from build123d import *

# Parameters (mm, degrees)
SKETCH_1_R               = 2.5
SKETCH_1_R_2             = 0.925
EXTRUDE_1_DEPTH          = 3
CUT_EXTRUDE_2_DEPTH      = 5.636809248
PATTERN_CIRCULAR_1_COUNT = 6
EXTRUDE_START            = 1
SKETCH_2_R               = 2.5
EXTRUDE_2_DEPTH          = 1
SKETCH_2_3_W             = 4
SKETCH_2_3_H             = 0.6
EXTRUDE_3_DEPTH          = 2
SKETCH_2_4_W             = 0.6
SKETCH_2_4_H             = 2.5
EXTRUDE_4_DEPTH          = 1


with BuildPart() as part:
    # 草图1 → 凸台-拉伸1 (new body)
    with BuildSketch(Plane.XY):
        Circle(SKETCH_1_R)
        Circle(SKETCH_1_R_2, mode=Mode.SUBTRACT)
    extrude(amount=EXTRUDE_1_DEPTH)

    # 草图1<3> → 切除-拉伸2 (cut, through all)
    with BuildSketch(Plane.XY):
        with BuildLine():
            Line((1.03720071, 0.442455292), (0.85081958, 0.362947713))
            ThreePointArc((0.85081958, 0.362947713), (0.906265169, 0.185225388), (0.925, 0))
            ThreePointArc((0.925, 0), (0.906265169, -0.185225388), (0.85081958, -0.362947713))
            Line((0.85081958, -0.362947713), (1.03720071, -0.442455292))
            add(Edge.make_bspline(
                [(1.03720071, -0.442455292), (1.04510701, -0.445828009), (1.067871965, -0.453596987), (1.113314547, -0.461522157), (1.188023144, -0.464138789), (1.284367459, -0.452433849), (1.404657298, -0.420054467), (1.538436606, -0.361310704), (1.660601931, -0.285147073), (1.748638649, -0.214154324), (1.79986288, -0.166729965), (1.818980117, -0.1481092)],
                knots=[0, 0, 0, 0, 0, 0.005604068, 0.015718248, 0.029959916, 0.048733667, 0.068727063, 0.096888892, 0.125050566, 0.14248965, 0.14248965, 0.14248965, 0.14248965, 0.14248965], degree=4))
            ThreePointArc((1.818980117, -0.1481092), (1.823494408, -0.074115744), (1.825, 0))
            ThreePointArc((1.825, 0), (1.823494408, 0.074115744), (1.818980117, 0.1481092))
            add(Edge.make_bspline(
                [(1.03720071, 0.442455292), (1.04510701, 0.445828009), (1.067871965, 0.453596987), (1.113314547, 0.461522157), (1.188023144, 0.464138789), (1.284367459, 0.452433849), (1.404657298, 0.420054467), (1.538436606, 0.361310704), (1.660601931, 0.285147073), (1.748638649, 0.214154324), (1.79986288, 0.166729965), (1.818980117, 0.1481092)],
                knots=[0, 0, 0, 0, 0, 0.005604068, 0.015718248, 0.029959916, 0.048733667, 0.068727063, 0.096888892, 0.125050566, 0.14248965, 0.14248965, 0.14248965, 0.14248965, 0.14248965], degree=4))
        make_face()
    cut_extrude_2 = extrude(amount=CUT_EXTRUDE_2_DEPTH, mode=Mode.SUBTRACT)

    # 阵列(圆周)1: 切除-拉伸2 ×6 about axis
    pattern_circular_1_axis = Axis((0, 0, 3), (0, 0, 1))
    for i in range(1, PATTERN_CIRCULAR_1_COUNT):
        add(cut_extrude_2.rotate(pattern_circular_1_axis, i * 360 / PATTERN_CIRCULAR_1_COUNT), mode=Mode.SUBTRACT)

    # 草图2 → 凸台-拉伸2 (add)
    with BuildSketch(Plane(origin=(0, 0, 0), x_dir=(-1, 0, 0), z_dir=(0, 0, -1)).offset(EXTRUDE_START)):
        Circle(SKETCH_2_R)
    extrude(amount=-EXTRUDE_2_DEPTH)

    # 草图2<3> → 凸台-拉伸3 (add)
    with BuildSketch(Plane(origin=(0, 0, 0), x_dir=(-1, 0, 0), z_dir=(0, 0, -1)).offset(EXTRUDE_START)):
        Rectangle(SKETCH_2_3_W, SKETCH_2_3_H)
    extrude(amount=EXTRUDE_3_DEPTH)

    # 草图2<4> → 凸台-拉伸4 (add)
    with BuildSketch(Plane(origin=(0, 0, 0), x_dir=(-1, 0, 0), z_dir=(0, 0, -1)).offset(EXTRUDE_START)):
        Rectangle(SKETCH_2_4_W, SKETCH_2_4_H)
    extrude(amount=EXTRUDE_4_DEPTH)


solid = part.part
Geometry: final body of the model. Coordinates: model frame, mm. A direction names the side the tool comes from. Round coordinates to 2 decimals unless told otherwise and drop trailing zeros. Loops run counter-clockwise (first coordinate to the right, second up) from the corner with the lowest first, then second, coordinate; pieces in that order, holes last. Notation, with made-up numbers: (73.25, 60.25) -> (91.25, 60.25) arc R22 cw to (91.25, 98.25) -> close; hole circle Ø8 at (3.25, 19.25). An arc over 180 degrees is marked (long way). One line per question, with ' | ' between items. Start each with the question number.
1. Mould query, pull axis X, two halves, no side actions, for faces 4 (the face through (0, -0.3, -2.2)), 5 (the face through (-0.3, 0.8, -1.5)), 6 (the face through (0, 0, 0)). Classes: pulls with the +X half, pulls with the -X half, needs draft (parallel to the pull), parting line crosses it, or undercut.
2. Contact query for flat-ended pins moving along their axis: pin 1 (0.8 mm diameter, centred on y = -1, z = -1.5, fed in from +X); pin 2 (1.6 mm diameter, centred on x = -1, z = -1.5, fed in from +Y); pin 3 (0.5 mm diameter, centred on y = 0, z = -1.5, fed in from +X). Output: stop coordinate, or through.
3. Set-up query: faces 1 (the face through (0.3, -0.8, -1.5)), 2 (the face through (-0.3, -0.8, -1.5)), 3 (the face through (0.3, 0.8, -1.5)). Return all of +Z, -Z, +X, -X, +Y, -Y with unobstructed straight access to the full face (end or side cutting, diameter ignored); none if empty.
4. Section A-A on x = 0. Output: boundary loops of the cut face in (y, z) (3 decimals).
5. Line query: line 1 along X through (y, z) = (1.25, 2); line 2 along Z through (x, y) = (-0.6, -1); line 3 along Z through (x, y) = (-1.4, -1.05). Output: solid intervals per line, ascending. Write a range as [from, to].
Returned:
1) face 4: needs draft | face 5: pulls with the -X half | face 6: undercut
2) pin 1: stops at x = 0.3 | pin 2: stops at y = 2.47 | pin 3: stops at x = 2
3) face 1: -Z, +X, -Y | face 2: -Z, -X, -Y | face 3: -Z, +X, +Y
4) outline: (-2.5, -1) -> (-1.25, -1) -> (-1.25, -2) -> (-0.3, -2) -> (-0.3, -3) -> (0.3, -3) -> (0.3, -2) -> (1.25, -2) -> (1.25, -1) -> (2.5, -1) -> (2.5, 3) -> (0.925, 3) -> (0.925, 0) -> (-0.925, 0) -> (-0.925, 3) -> (-2.5, 3) -> close
5) line 1: x = [-2.17, -1.08], [-0.19, 0.19], [1.08, 2.17] | line 2: z = [-1, 0] | line 3: z = [-1, 3]
